The model under review builds one solid part; all positions refer to its coordinate system, in mm. A direction names the side the tool comes from. Coordinates: 2 decimals unless noted, no trailing zeros. Order: outer loops, then holes, each group sorted by start corner. A loop starts at its lowest first (then second) coordinate and runs counter-clockwise, first axis right, second up. Notation, with made-up numbers: M 63.5,86.25 L 106.5,86.25 A23 cw 106.5,104.25 Z; hole C 38.25,-13 d6. An arc over 180 degrees is marked long. One line per item, written item: value.
Autodesk Inventor part; units mm, degrees
ref_plane "YZ Plane" through (0, 0, 0) normal (1, 0, 0) x (0, 1, 0)
ref_plane "XZ Plane" through (0, 0, 0) normal (0, 1, 0) x (-1, 0, 0)
ref_plane "XY Plane" through (0, 0, 0) normal (0, 0, 1) x (1, 0, 0)
sketch "Sketch1" plane through (0, 0, 0) normal (0, 0, 1) x (1, 0, 0)
  circle A0 centre (0, 0) radius 12.5
  line L0 (-43.5003, 20.018) -> (43.5003, 20.018)
  line L1 (43.5003, 20.018) -> (43.5003, -20.018)
  line L2 (43.5003, -20.018) -> (-43.5003, -20.018)
  line L3 (-43.5003, -20.018) -> (-43.5003, 20.018) construction
  line L4 (-43.5003, 20.018) -> (43.5003, -20.018) construction
  line L5 (43.5003, 20.018) -> (-43.5003, -20.018) construction
  line L6 (7.8932, 9.6927) -> (7.8932, 20.018)
  line L7 (-6.4997, -10.6772) -> (-6.4997, -20.018)
  circle A1 centre (37.5003, 10.982) radius 3.5 construction
  circle A2 centre (37.5003, -14.018) radius 3.5 construction
  circle A3 centre (37.5003, 10.982) radius 3
  circle A4 centre (37.5003, -14.018) radius 3
  dimension "d0" = 25
  dimension "d6" = 50
  dimension "d7" = 6
  dimension "d8" = 6
  dimension "d9" = 6
  dimension "d10" = 6
extrude "Extrusion1" add sketch "Sketch1" along normal blind 3 contours A0 L6 L0 L1 L2 L7
fillet "Fillet1" radius 4 4 edges at (43.5003, -20.018, 1.5) (43.5003, 20.018, 1.5) (-6.4997, -20.018, 1.5) (7.8932, 20.018, 1.5)
properties part number "domePlaceSingle"
(1) We need section B-B, the plane x = 8.5. State the section outline as (y, z) points.
Geometry results:
outline: M -20.02,0 L -9.17,0 L -9.17,3 L -20.02,3 Z; M 9.17,0 L 18.14,0 L 18.14,3 L 9.17,3 Z
(2) Insertion check: pin 1 Ø1.5 at (y, z) = (13, 1) entering from -X; pin 2 Ø1 at (y, z) = (-3, 0.5) entering from -X; pin 3 Ø3.5 at (x, y) = (37.5, 10.98) entering from -Z. Each pin has a flat end and moves straight along its axis. Give the tip position at first contact, or say it passes through.
Geometry results:
pin 1: stops at x = 7.89
pin 2: stops at x = 12
pin 3: passes through
(3) We need section A-A, the plane y = 12.5. State the section outline as (x, z) points, plus the area to 3 significant figures.
Geometry results:
outline: M 7.89,0 L 34.91,0 L 34.91,3 L 7.89,3 Z; M 40.09,0 L 43.5,0 L 43.5,3 L 40.09,3 Z
area: 91.3 mm2
(4) We need section D-D, the plane y = -6. State the section outline as (x, z) points.
Geometry results:
outline: M 10.97,0 L 43.5,0 L 43.5,3 L 10.97,3 Z
(5) We need section C-C, the plane z = 1.8. State the section outline as (x, y) points, plus the area to 3 significant figures.
Geometry results:
outline: M -6.5,-16.02 A4 ccw -2.5,-20.02 L 39.5,-20.02 A4 ccw 43.5,-16.02 L 43.5,16.02 A4 ccw 39.5,20.02 L 11.89,20.02 A4 ccw 7.89,16.02 L 7.89,9.69 A12.5 cw -6.5,-10.68 Z; hole C 37.5,-14.02 d6; hole C 37.5,10.98 d6
area: 1,410 mm2
(6) Mouldability with a two-part tool opening along X and no side actions: class faces 3 (the cylindrical face through (40.36, 10.08, 1.48)), 4 (the cylindrical face through (9.1, 18.88, 1.52)), 5 (the flat face through (43.5, 0, 1)), 6 (the cylindrical face through (40.36, -14.92, 1.48)) as +X half, -X half, draft (parallel to the pull), parting line (faces both ways), or undercut.
Geometry results:
face 3: undercut
face 4: -X half
face 5: +X half
face 6: undercut
(7) Tool access review of faces 1 (the flat face through (7.893, 13, 1)), 2 (the flat face through (26, 20.018, 1)): name each direction out of +Z, -Z, +X, -X, +Y, -Y from which nothing blocks a thin tool from reaching the whole face with its end or side.
Geometry results:
face 1: +Z, -Z, -X, +Y
face 2: +Z, -Z, +X, -X, +Y
(8) For L1, parallel to Y at x = 39, z = 2.4; L2, parallel to Y at x = 38, z = 1.9; L3, parallel to X at y = -13.5, z = 0.4, list the stretches that pass through material, from the lowest coordinate up.
Geometry results:
L1: y = -20.02 to -16.62, -11.42 to 8.38, 13.58 to 20.02
L2: y = -20.02 to -16.98, -11.06 to 8.02, 13.94 to 20.02
L3: x = -6.5 to 34.55, 40.46 to 43.5
